Check sheet for the modelled part. Datum: model origin and axes. Units: mm. Face numbers are marked on the shaded views. Round coordinates to 2 decimals unless told otherwise and drop trailing zeros. Write each loop counter-clockwise with the first axis right and the second up, starting at its lowest first coordinate (ties: lowest second). Pieces come first, ordered by that corner, then holes. Notation, with made-up numbers: (44, 73.5) -> (89, 73.5) arc R24 ccw to (89, 85.5) -> close; hole circle Ø5 at (45, -3). An arc over 180 degrees is marked (long way). Write item = value, one per line.
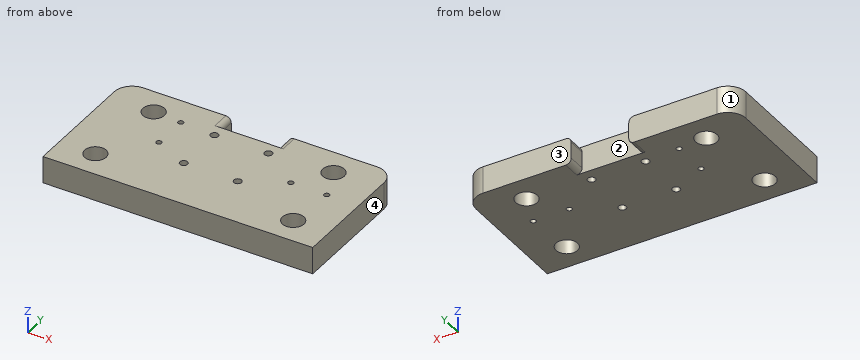
from build123d import *

# Parameters (mm, degrees)
SKETCH_1_R          = 2.15
EXTRUDE_1_DEPTH     = 15
SKETCH_2_R          = 6
CUT_EXTRUDE_1_DEPTH = 86.183625187
FILLET_1_R          = 3
SKETCH_3_R          = 1.5
CUT_EXTRUDE_2_DEPTH = 86.183625187
SKETCH_4_R          = 1.5
CUT_EXTRUDE_3_DEPTH = 86.183625187


with BuildPart() as part:
    # 草图1 → 凸台-拉伸1 (new body)
    with BuildSketch(Plane.XY):
        with BuildLine():
            Line((16, 37.5), (65, 37.5))
            ThreePointArc((65, 37.5), (72.071067812, 34.571067812), (75, 27.5))
            Line((75, 27.5), (75, -37.5))
            Line((75, -37.5), (-75, -37.5))
            Line((-75, -37.5), (-75, 27.5))
            ThreePointArc((-75, 27.5), (-72.071067812, 34.571067812), (-65, 37.5))
            Line((-65, 37.5), (-16, 37.5))
            Line((-16, 37.5), (-16, 27.5))
            Line((-16, 27.5), (16, 27.5))
            Line((16, 27.5), (16, 37.5))
        make_face()
        with Locations((-15, 20.5)):
            Circle(SKETCH_1_R, mode=Mode.SUBTRACT)
        with Locations((15, 20.5)):
            Circle(SKETCH_1_R, mode=Mode.SUBTRACT)
        with Locations((-15, -7.5)):
            Circle(SKETCH_1_R, mode=Mode.SUBTRACT)
        with Locations((15, -7.5)):
            Circle(SKETCH_1_R, mode=Mode.SUBTRACT)
    extrude(amount=EXTRUDE_1_DEPTH)

    # 草图2 → 切除-拉伸1 (cut, through all)
    with BuildSketch(Plane.XY.offset(15)):
        with Locations((-50, 22.5)):
            Circle(SKETCH_2_R)
        with Locations((50, 22.5)):
            Circle(SKETCH_2_R)
        with Locations((-55, -22.5)):
            Circle(SKETCH_2_R)
        with Locations((55, -22.5)):
            Circle(SKETCH_2_R)
    extrude(amount=-CUT_EXTRUDE_1_DEPTH, mode=Mode.SUBTRACT)

    # 圆角1
    fillet_1_edges = [part.edges().sort_by_distance(p)[0] for p in [
        (-16, 32.5, 15),
        (16, 32.5, 0),
        (-16, 32.5, 0),
        (16, 32.5, 15),
    ]]
    fillet(fillet_1_edges, radius=FILLET_1_R)

    # 草图3 → 切除-拉伸2 (cut, through all)
    with BuildSketch(Plane.XY.offset(15)):
        with Locations((-34.29, 1.5)):
            Circle(SKETCH_3_R)
        with Locations((-34.29, 21.5)):
            Circle(SKETCH_3_R)
    extrude(amount=-CUT_EXTRUDE_2_DEPTH, mode=Mode.SUBTRACT)

    # 草图4 → 切除-拉伸3 (cut, through all)
    with BuildSketch(Plane.XY.offset(15)):
        with Locations((57.21, 4.5)):
            Circle(SKETCH_4_R)
        with Locations((37.21, 4.5)):
            Circle(SKETCH_4_R)
    extrude(amount=-CUT_EXTRUDE_3_DEPTH, mode=Mode.SUBTRACT)


solid = part.part
(1) Go/stop test with flat-tipped pins: P1, Ø7, axis at y = 32.5, z = 9.5, coming from the -X side; P2, Ø4.5, axis at x = -2, z = 5.5, coming from the +Y side. Record where each tip stops, or that it passes through.
Worked answers:
P1 = -74.89
P2 = 27.5
(2) Material ranges on L1, parallel to Y at x = -15, z = 10; L2, parallel to Y at x = 37, z = 1.5; L3, parallel to Y at x = -34.29, z = 4.5, recorded low to high. Write a range as [from, to].
Worked answers:
L1 = [-37.5, -9.65], [-5.35, 18.35], [22.65, 27.5]
L2 = [-37.5, 3.01], [5.99, 37.5]
L3 = [-37.5, 0], [3, 20], [23, 37.5]
(3) Sectioned sample at B-B on x = -51.5. Enter the section's corners in (y, z).
Worked answers:
outline = (-37.5, 0) -> (-27.37, 0) -> (-27.37, 15) -> (-37.5, 15) -> close; (-17.63, 0) -> (16.69, 0) -> (16.69, 15) -> (-17.63, 15) -> close; (28.31, 0) -> (37.5, 0) -> (37.5, 15) -> (28.31, 15) -> close
(4) Sectioned sample at D-D on x = 46. Enter the section's corners in (y, z), then the cut area to 3 significant figures.
Worked answers:
outline = (-37.5, 0) -> (18.03, 0) -> (18.03, 15) -> (-37.5, 15) -> close; (26.97, 0) -> (37.5, 0) -> (37.5, 15) -> (26.97, 15) -> close
area = 991 mm²
(5) Sectioned sample at A-A on z = 8.75. Count the separate pieces of the cut face and the enclosed holes in it, then the cut area to 3 significant figures.
Worked answers:
separate_pieces = 1
enclosed_holes = 12
area = 10,300 mm²
(6) Sectioned sample at C-C on y = -7.5. Enter the section's corners in (x, z), then the cut area to 3 significant figures.
Worked answers:
outline = (-75, 0) -> (-17.15, 0) -> (-17.15, 15) -> (-75, 15) -> close; (-12.85, 0) -> (12.85, 0) -> (12.85, 15) -> (-12.85, 15) -> close; (17.15, 0) -> (75, 0) -> (75, 15) -> (17.15, 15) -> close
area = 2,120 mm²
(7) Release check for a two-part mould opening along X. For the marked faces 1, 2, 3 and 4 record: pulls with the +X half, pulls with the -X half, needs draft (parallel to the pull), parting line crosses it, or undercut.
Worked answers:
face_1 = pulls with the -X half
face_2 = undercut
face_3 = needs draft
face_4 = pulls with the +X half
